Input: dimensioned drawing with shaded views. Units: mm. Origin: part minimum x, y, z. A direction names the side the tool comes from. Coordinates: 2 decimals unless noted, no trailing zeros. Order: outer loops, then holes, each group sorted by start corner. A loop starts at its lowest first (then second) coordinate and runs counter-clockwise, first axis right, second up. Notation, with made-up numbers: M 68,-21.75 L 105,-21.75 A18 ccw 105,-17.75 Z; hole C 21.25,58.25 d5. An arc over 180 degrees is marked long. Use CSV: the item, a comma, the result in double quotes. Start each with the question number.
1. Section query B-B on x = 16. Return the cut outline in (y, z).
2. Section query C-C on z = 10.5. Return the cut outline in (x, y).
3. Section query A-A on y = 1.5. Return the cut outline in (x, z).
4. First-contact query: P1, Ø1.5, axis at x = 44.5, y = 1.5, coming from the -Z side; P2, Ø5, axis at y = 6.5, z = 19.5, coming from the -X side; P3, Ø11, axis at x = 22.5, z = 99.5, coming from the +Y side. Flat tips, straight axial feed; report the tip coordinate or a pass-through.
5. Material intervals for line 1 (X direction, y = 4.25, z = 95); line 2 (Z direction, x = 45.5, y = 2.75); line 3 (Y direction, x = 28, z = 98), sorted ascending.
6. Set-up query: the marked faces 1 and 2. Return all of +Z, -Z, +X, -X, +Y, -Y with unobstructed straight access to the full face (end or side cutting, diameter ignored); none if empty.
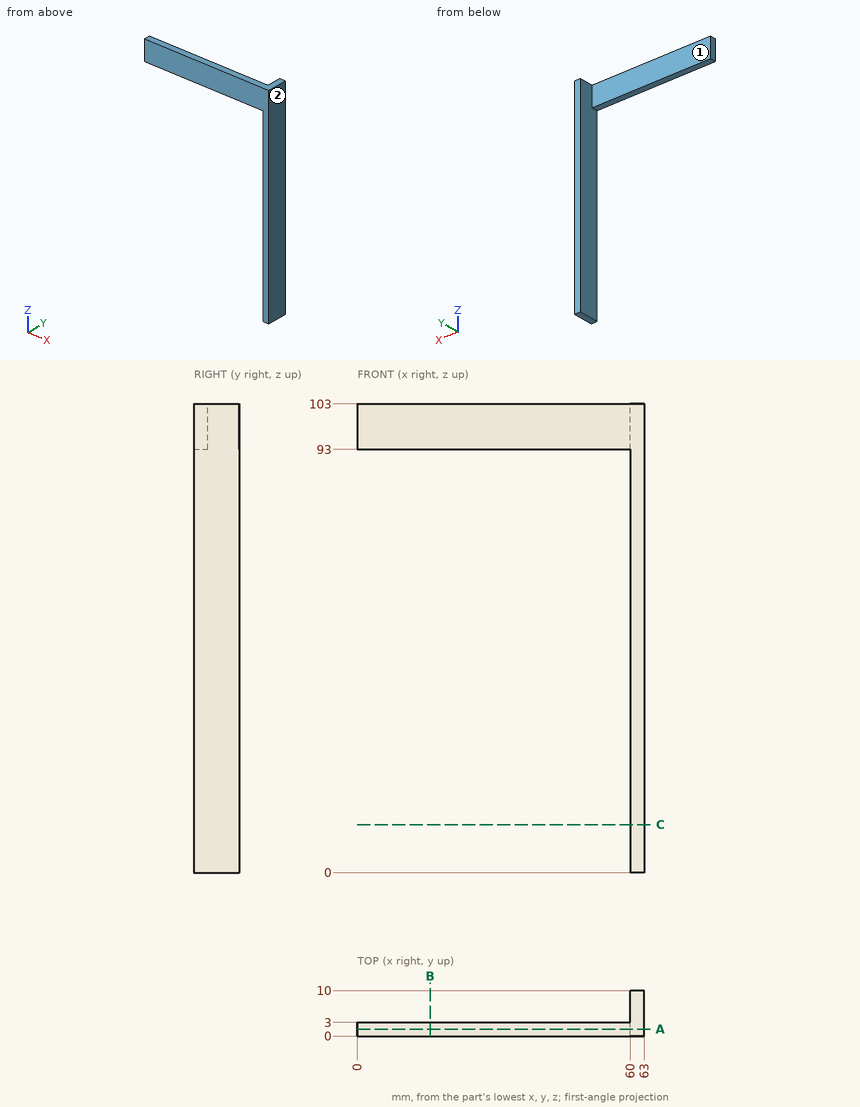
Results list:
1,outline,"M 0,93 L 3,93 L 3,103 L 0,103 Z"
2,outline,"M 60,0 L 63,0 L 63,10 L 60,10 Z"
3,outline,"M 0,93 L 60,93 L 60,0 L 63,0 L 63,103 L 0,103 Z"
4,P1,"stops at z = 93"
4,P2,"stops at x = 60"
4,P3,"stops at y = 3"
5,line 1,"x = 60 to 63"
5,line 2,"z = 93 to 103"
5,line 3,"y = 0 to 3"
6,face 1,"+Z, -Z, -X, +Y"
6,face 2,"+Z, -Z, +X, +Y, -Y"
